```python
from build123d import *

# Parameters (mm, degrees)
SKETCH1_W           = 40
SKETCH1_H           = 30
BOSS_EXTRUDE1_DEPTH = 50
SKETCH2_W           = 30
SKETCH2_H           = 45
CUT_EXTRUDE1_DEPTH  = 30
FILLET1_R           = 10
SKETCH3_R           = 1.984375
CUT_EXTRUDE2_DEPTH  = 30
SKETCH4_R           = 3.083104926
CUT_EXTRUDE3_DEPTH  = 55
SKETCH5_R           = 1.984375
CUT_EXTRUDE4_DEPTH  = 30


with BuildPart() as part:
    # Sketch1 → Boss-Extrude1 (new body)
    with BuildSketch(Plane(origin=(0, 0, 0), x_dir=(1, 0, 0), z_dir=(0, 1, 0))):
        with Locations((20, 15)):
            Rectangle(SKETCH1_W, SKETCH1_H)
    extrude(amount=BOSS_EXTRUDE1_DEPTH)

    # Sketch2 → Cut-Extrude1 (cut)
    with BuildSketch(Plane.XY):
        with Locations((20, 27.5)):
            Rectangle(SKETCH2_W, SKETCH2_H)
    extrude(amount=-CUT_EXTRUDE1_DEPTH, mode=Mode.SUBTRACT)

    # Fillet1
    fillet1_edges = [part.edges().sort_by_distance(p)[0] for p in [
        (37.5, 50, -30),
        (37.5, 50, 0),
        (2.5, 50, -30),
        (2.5, 50, 0),
    ]]
    fillet(fillet1_edges, radius=FILLET1_R)

    # Sketch3 → Cut-Extrude2 (cut)
    with BuildSketch(Plane(origin=(0, 5, 0), x_dir=(1, 0, 0), z_dir=(0, 1, 0))):
        with Locations((10.272803798, 5)):
            Circle(SKETCH3_R)
        with Locations((10.272803798, 25)):
            Circle(SKETCH3_R)
    extrude(amount=-CUT_EXTRUDE2_DEPTH, mode=Mode.SUBTRACT)

    # Sketch4 → Cut-Extrude3 (cut)
    with BuildSketch(Plane(origin=(40, 0, 0), x_dir=(0, 0, -1), z_dir=(1, 0, 0))):
        with Locations((15, 40)):
            Circle(SKETCH4_R)
    extrude(amount=-CUT_EXTRUDE3_DEPTH, mode=Mode.SUBTRACT)

    # Sketch5 → Cut-Extrude4 (cut)
    with BuildSketch(Plane(origin=(0, 5, 0), x_dir=(1, 0, 0), z_dir=(0, 1, 0))):
        with Locations((30, 25)):
            Circle(SKETCH5_R)
        with Locations((30, 5)):
            Circle(SKETCH5_R)
    extrude(amount=-CUT_EXTRUDE4_DEPTH, mode=Mode.SUBTRACT)


solid = part.part
```
CAD build for the part. Positions are in the model's coordinates, mm. A direction names the side the tool comes from. Round coordinates to 2 decimals unless told otherwise and drop trailing zeros. Write each loop counter-clockwise with the first axis right and the second up, starting at its lowest first coordinate (ties: lowest second). Pieces come first, ordered by that corner, then holes. Notation, with made-up numbers: (68, -8) - (73, -8) arc R14 cw to (73, -2) - close; hole circle Ø5 at (-26, 44). An arc over 180 degrees is marked (long way). Return JSON: item names as keys, results as strings. Group by question number.
Item 1: Mould opens along X. For faces 3 (the face through (0, 25, -15)), 4 (the face through (35, 27, -15)), 5 (the face through (2.53, 36.99, -14.33)) say: +X half, -X half, draft (parallel to the pull), parting line (faces both ways), or undercut.
Item 2: Band-saw the part on C-C on y = 15. List the corners of the cut face in (x, z), plus the area to 3 significant figures.
Item 3: Band-saw the part on D-D on x = 36.5. List the corners of the cut face in (y, z).
Item 4: Flat gauge pins, fed straight in: pin 1 Ø10 at (x, y) = (6, 11) entering from +Z; pin 2 Ø6.5 at (x, z) = (30, -5) entering from +Y; pin 3 Ø10 at (x, z) = (32, -5) entering from +Y. Where does each tip first touch, or does it go through?
Item 5: Band-saw the part on A-A on x = 30. List the corners of the cut face in (y, z), plus the area to 3 significant figures.
Item 6: Probe probe 1 along X at (y, z) = (2.85, -5); probe 2 along Z at (x, y) = (30, 1); probe 3 along X at (y, z) = (17, -13.25). List the from-to ranges inside material, lowest first.
Item 7: Band-saw the part on B-B on z = -15. List the corners of the cut face in (x, y).
Item 8: 3-axis set-ups, long thin cutter, end or side, ignore diameter. For faces 1 (the face through (5, 27, -15)), 2 (the face through (37.53, 36.99, -14.33)): which of +Z, -Z, +X, -X, +Y, -Y reach the whole face in a straight line?
Resolved:
{
 "1": {"face 3": "-X half", "face 4": "undercut", "face 5": "draft"},
 "2": {"outline": "(0, -30) - (5, -30) - (5, 0) - (0, 0) - close; (35, -30) - (40, -30) - (40, 0) - (35, 0) - close", "area": "300 mm²"},
 "3": {"outline": "(0, -30) - (40, -30) arc R10 ccw to (50, -20) - (50, -10) arc R10 ccw to (40, 0) - (0, 0) - close; hole circle Ø6.17 at (40, -15)"},
 "4": {"pin 1": "stops at z = 0", "pin 2": "stops at y = 5", "pin 3": "stops at y = 49.95"},
 "5": {"outline": "(0, -30) - (5, -30) - (5, -26.98) - (0, -26.98) - close; (0, -23.02) - (5, -23.02) - (5, -6.98) - (0, -6.98) - close; (0, -3.02) - (5, -3.02) - (5, 0) - (0, 0) - close", "area": "110 mm²"},
 "6": {"probe 1": "x = 0 to 8.29, 12.26 to 28.02, 31.98 to 40", "probe 2": "z = -30 to -26.98, -23.02 to -6.98, -3.02 to 0", "probe 3": "x = 0 to 5, 35 to 40"},
 "7": {"outline": "(0, 0) - (40, 0) - (40, 36.92) - (35, 36.92) - (35, 5) - (5, 5) - (5, 36.92) - (0, 36.92) - close; (0, 43.08) - (5, 43.08) - (5, 50) - (0, 50) - close; (35, 43.08) - (40, 43.08) - (40, 50) - (35, 50) - close"},
 "8": {"face 1": "+Z, -Z, +Y", "face 2": "+X, -X"}
}
